Read the model definition and answer for the solid it produces. Units are mm, in the model's axes. A direction names the side the tool comes from. Round coordinates to 2 decimals unless told otherwise and drop trailing zeros. Write each loop counter-clockwise with the first axis right and the second up, starting at its lowest first coordinate (ties: lowest second). Pieces come first, ordered by that corner, then holes. Notation, with made-up numbers: (34.5, 38.25) -> (77.5, 38.25) arc R21 ccw to (77.5, 70.25) -> close; hole circle Ø7 at (52, -18.75). An arc over 180 degrees is marked (long way). Return JSON: item names as keys, results as strings. Group by question number.
(1) A cutting plane is placed at C-C on y = 55. Give the vertices of the cut face in (x, z).
(2) For faces 5 (the cylindrical face through (7.01, -1.48, -4.8)), 6 (the flat face through (0, 0, 5)), determine the directions among +Z, -Z, +X, -X, +Y, -Y from which every point of the face is accessible in a straight line to the end or side of a thin tool.
(3) A cutting plane is placed at B-B on z = 0. Give the vertices of the cut face in (x, y), then the cut area to 3 significant figures.
(4) A cutting plane is placed at D-D on z = -8.75. Give the vertices of the cut face in (x, y), then the cut area to 3 significant figures.
(5) Given pin 1 (2 mm diameter, centred on y = 64, z = 3, fed in from -X); pin 2 (4 mm diameter, centred on x = 5.66, z = -5.66, fed in from +Y); pin 3 (5 mm diameter, centred on x = -3, y = 17, fed in from +Z), each flat-ended and moving along its own axis, determine where each tip first touches the part or whether it passes through.
(6) A cutting plane is placed at A-A on x = 0. Give the vertices of the cut face in (y, z), then the cut area to 3 significant figures.
(7) The mould has two halves that part along X. Classify faces 1 (the cylindrical face through (1.352, 49.3, 4.292)), 2 (the flat face through (0, 100, 0)), 3 (the cylindrical face through (-7.076, -1.479, 6.395)), 4 (the cylindrical face through (-7.076, -1.479, -4.919)): released by +X, released by -X, zero draft, split by the parting line, or undercut.
(8) Straight lines are drawn through the part: line 1 (Y direction, x = -3, z = 11); line 2 (X direction, y = 87.5, z = -3.75); line 3 (X direction, y = 25, z = -1.5). For each, find the intervals that lie inside material, in ascending order.
```python
from build123d import *

# Parameters (mm, degrees)
SKETCH_1_R          = 12
EXTRUDE_2_DEPTH     = 3
SKETCH_2_R          = 1.6
CUT_EXTRUDE_1_DEPTH = 3
SKETCH_3_R          = 4.5
EXTRUDE_3_DEPTH     = 100


with BuildPart() as part:
    # 草图1 → 凸台-拉伸2 (new body)
    with BuildSketch(Plane(origin=(0, 0, 0), x_dir=(1, 0, 0), z_dir=(0, 1, 0))):
        with Locations(Location((0, 0, 0), (0, 0, 270))):
            Circle(SKETCH_1_R)
    extrude(amount=-EXTRUDE_2_DEPTH)

    # 草图2 → 切除-拉伸1 (cut)
    with BuildSketch(Plane(origin=(0, 0, 0), x_dir=(1, 0, 0), z_dir=(0, 1, 0))):
        with Locations(Location((5.656854249, -5.656854249, 0), (0, 0, 270))):
            Circle(SKETCH_2_R)
        with Locations(Location((-5.656854249, -5.656854249, 0), (0, 0, 270))):
            Circle(SKETCH_2_R)
        with Locations(Location((-5.656854249, 5.656854249, 0), (0, 0, 270))):
            Circle(SKETCH_2_R)
        with Locations(Location((5.656854249, 5.656854249, 0), (0, 0, 270))):
            Circle(SKETCH_2_R)
    extrude(amount=-CUT_EXTRUDE_1_DEPTH, mode=Mode.SUBTRACT)

    # 草图3 → 凸台-拉伸3 (add)
    with BuildSketch(Plane(origin=(0, 0, 0), x_dir=(1, 0, 0), z_dir=(0, 1, 0))):
        with Locations(Location((0, 0, 0), (0, 0, 270))):
            Circle(SKETCH_3_R)
    extrude(amount=EXTRUDE_3_DEPTH)


solid = part.part
```
Checks:
{
 "1": {"outline": "circle Ø9 at (0, 0)"},
 "2": {"face 5": "+Y, -Y", "face 6": "+Y"},
 "3": {"outline": "(-12, -3) -> (12, -3) -> (12, 0) -> (4.5, 0) -> (4.5, 100) -> (-4.5, 100) -> (-4.5, 0) -> (-12, 0) -> close", "area": "972 mm^2"},
 "4": {"outline": "(-8.21, -3) -> (8.21, -3) -> (8.21, 0) -> (-8.21, 0) -> close", "area": "49.3 mm^2"},
 "5": {"pin 1": "stops at x = -4.03", "pin 2": "stops at y = 0", "pin 3": "stops at z = 4.47"},
 "6": {"outline": "(-3, -12) -> (0, -12) -> (0, -4.5) -> (100, -4.5) -> (100, 4.5) -> (0, 4.5) -> (0, 12) -> (-3, 12) -> close", "area": "972 mm^2"},
 "7": {"face 1": "split by the parting line", "face 2": "zero draft", "face 3": "undercut", "face 4": "undercut"},
 "8": {"line 1": "y = -3 to 0", "line 2": "x = -2.49 to 2.49", "line 3": "x = -4.24 to 4.24"}
}
